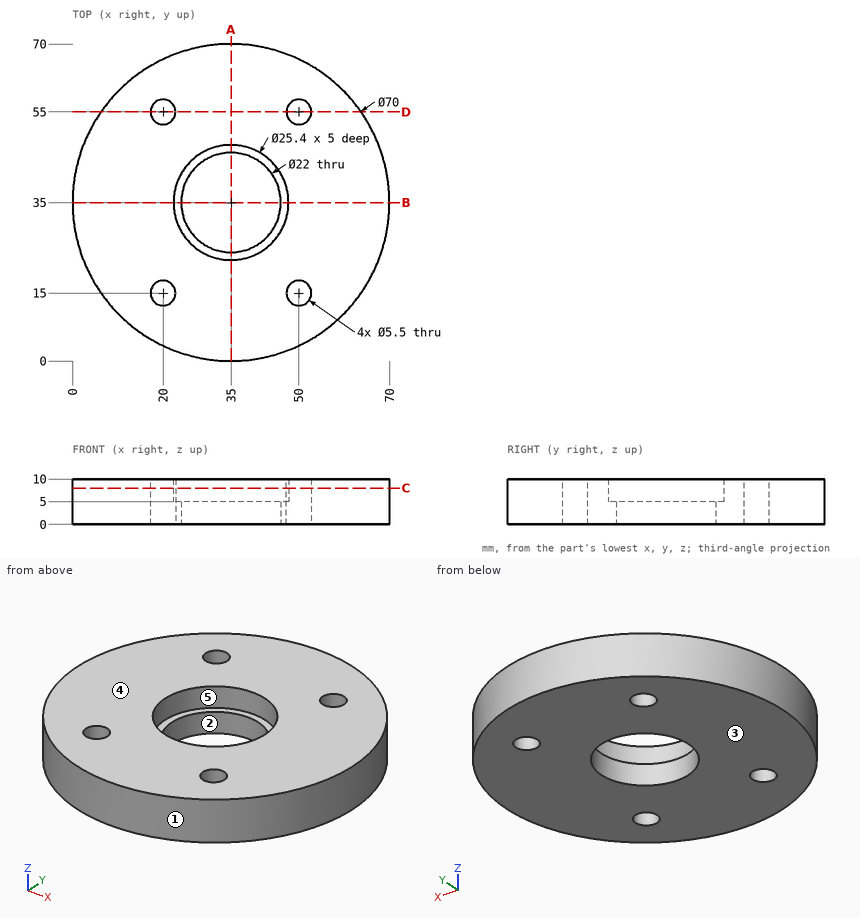
The drawing under review shows one solid part. Ordinate dimensions are in mm from its lowest x, y, z. A direction names the side the tool comes from. Give positions to 0.01 mm unless a question says otherwise; leave off trailing zeros. Order: outer loops, then holes, each group sorted by start corner. A loop starts at its lowest first (then second) coordinate and runs counter-clockwise, first axis right, second up. Notation, with made-up numbers: (8, 7.5) - (57, 7.5) arc R19 ccw to (57, 32.5) - close; hole circle Ø6 at (35.5, -21.5). An arc over 180 degrees is marked (long way). Answer as a JSON object with one key per item and string values. Group by question number.
Item 1: Take a section at D-D on y = 55. Give the boundary of the cut face in (x, z).
Item 2: Clearance check with flat-ended pins moving along their axes: pin 1 Ø2 at (y, z) = (23, 6.5) entering from +X; pin 2 Ø1 at (x, z) = (14.5, 1.5) entering from +Y; pin 3 Ø5 at (y, z) = (51, 7) entering from -X. State where each tip first meets the part, or that it passes through.
Item 3: Take a section at A-A on x = 35. Give the boundary of the cut face in (y, z), and give its area (3 significant figures).
Item 4: Draft analysis for pull direction Y (two halves, no side actions). For the marked faces 1, 2 and 3, state which applies: pulls with the +Y half, pulls with the -Y half, needs draft (parallel to the pull), parting line crosses it, or undercut.
Item 5: Machinability: for the marked faces 4 and 5, which of the approach directions +Z, -Z, +X, -X, +Y, -Y give a long, thin tool a straight path to every point of the face, cutting with its end or side? Answer none if there is none.
Item 6: Wall thickness on line 1 along Y through (x, z) = (35, 1.2); line 2 along Y through (x, z) = (20, 2.75); line 3 along Y through (x, z) = (31.5, 0.5): over which ranges is each line inside the solid? List them lowest first.
Item 7: Take a section at C-C on z = 8. Give the boundary of the cut face in (x, y).
Reported:
{
 "1": {"outline": "(6.28, 0) - (17.25, 0) - (17.25, 10) - (6.28, 10) - close; (22.75, 0) - (47.25, 0) - (47.25, 10) - (22.75, 10) - close; (52.75, 0) - (63.72, 0) - (63.72, 10) - (52.75, 10) - close"},
 "2": {"pin 1": "x = 68.23", "pin 2": "y = 63.72", "pin 3": "x = 2.71"},
 "3": {"outline": "(0, 0) - (24, 0) - (24, 5) - (22.3, 5) - (22.3, 10) - (0, 10) - close; (46, 0) - (70, 0) - (70, 10) - (47.7, 10) - (47.7, 5) - (46, 5) - close", "area": "463 mm^2"},
 "4": {"face 1": "parting line crosses it", "face 2": "undercut", "face 3": "needs draft"},
 "5": {"face 4": "+Z, +X, -X, +Y, -Y", "face 5": "+Z"},
 "6": {"line 1": "0 to 24, 46 to 70", "line 2": "3.38 to 12.25, 17.75 to 52.25, 57.75 to 66.62", "line 3": "0.18 to 24.57, 45.43 to 69.82"},
 "7": {"outline": "circle Ø70 at (35, 35); hole circle Ø5.5 at (20, 15); hole circle Ø5.5 at (20, 55); hole circle Ø25.4 at (35, 35); hole circle Ø5.5 at (50, 15); hole circle Ø5.5 at (50, 55)"}
}
